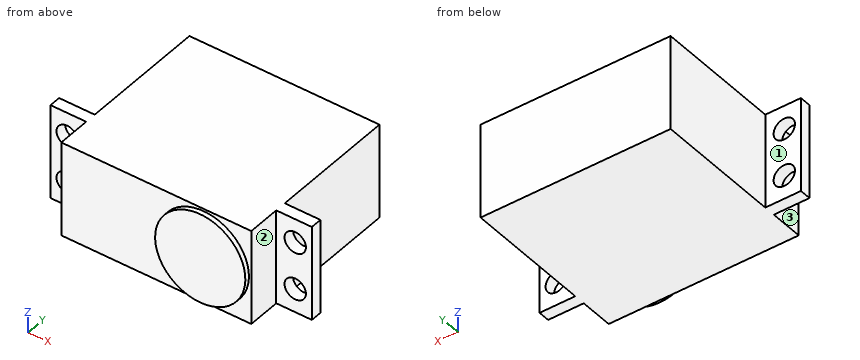
from build123d import *

# Parameters (mm, degrees)
SKETCH1_W            = 40
SKETCH1_H            = 20
BOSS_EXTRUDE1_DEPTH  = 36
SKETCH2_W            = 55
SKETCH2_H            = 20
BOSS_EXTRUDE2_DEPTH  = 2.4
M4_CLEARANCE_HOLE1_D = 4.5
SKETCH5_R            = 9.5
BOSS_EXTRUDE3_DEPTH  = 1


with BuildPart() as part:
    # Sketch1 → Boss-Extrude1 (new body)
    with BuildSketch(Plane(origin=(0, 0, 0), x_dir=(1, 0, 0), z_dir=(0, 1, 0))):
        Rectangle(SKETCH1_W, SKETCH1_H)
    extrude(amount=BOSS_EXTRUDE1_DEPTH)

    # Sketch2 → Boss-Extrude2 (add)
    with BuildSketch(Plane(origin=(0, 7, 0), x_dir=(1, 0, 0), z_dir=(0, 1, 0))):
        Rectangle(SKETCH2_W, SKETCH2_H)
    extrude(amount=BOSS_EXTRUDE2_DEPTH)

    # M4 Clearance Hole1 (through all)
    with Locations(Plane(origin=(0, 7, 0), x_dir=(-1, 0, 0), z_dir=(0, -1, 0))):
        with Locations((-24, 5), (-24, -5)):
            m4_clearance_hole1 = Hole(M4_CLEARANCE_HOLE1_D / 2)

    # Mirror1: M4 Clearance Hole1 across plane
    add(m4_clearance_hole1.mirror(Plane(origin=(0, 0, 0), x_dir=(0, 0, 1), z_dir=(1, 0, 0))), mode=Mode.SUBTRACT)

    # Sketch5 → Boss-Extrude3 (add)
    with BuildSketch(Plane.XZ):
        with Locations(Location((10, 0, 0), (0, 0, 270))):
            Circle(SKETCH5_R)
    extrude(amount=BOSS_EXTRUDE3_DEPTH)


solid = part.part
For this review, take the finished solid that the model builds, in its own axes (mm). Face numbers are marked on the shaded views. A direction names the side the tool comes from. Give positions to 0.01 mm unless a question says otherwise; leave off trailing zeros. Loops run counter-clockwise (first coordinate to the right, second up) from the corner with the lowest first, then second, coordinate; pieces in that order, holes last. Notation, with made-up numbers: M -22,-1.75 L 32,-1.75 A22 ccw 32,5.25 Z; hole C 80,51.5 d3. An arc over 180 degrees is marked long. Put each result on its own line as item: value. Start each with the question number.
(1) Add section C-C, the plane z = 0.25. Write out the cut boundary in (x, y).
(2) Add section A-A, the plane x = -24. Write out the cut boundary in (y, z).
(3) For pin 1 (1 mm diameter, centred on y = 30.5, z = -3.5, fed in from -X); pin 2 (6 mm diameter, centred on x = 24.5, z = 3, fed in from +Y); pin 3 (3.5 mm diameter, centred on x = 24, z = 5, fed in from +Y); pin 4 (8 mm diameter, centred on y = 20, z = 3, fed in from +X), all flat-tipped, find the tip position at first contact; note any pin that passes through.
(4) Machinability: for the marked faces 1, 2 and 3, which of the approach directions +Z, -Z, +X, -X, +Y, -Y give a long, thin tool a straight path to every point of the face, cutting with its end or side? Answer none if there is none.
(5) Add section B-B, the plane z = -5. Write out the cut boundary in (x, y).
(6) Add section D-D, the plane y = 21.5. Write out the cut boundary in (x, z), then the cut area to 3 significant figures.
(7) Wall thickness on L1, parallel to Z at x = -24, y = 8.3; L2, parallel to Y at x = -4, z = 2; L3, parallel to Y at x = 22.5, z = 8.75: over which ranges is each line inside the solid? List them lowest first.
Result:
1. outline: M -27.5,7 L -20,7 L -20,0 L 0.5,0 L 0.5,-1 L 19.5,-1 L 19.5,0 L 20,0 L 20,7 L 27.5,7 L 27.5,9.4 L 20,9.4 L 20,36 L -20,36 L -20,9.4 L -27.5,9.4 Z
2. outline: M 7,-10 L 9.4,-10 L 9.4,-7.25 L 7,-7.25 Z; M 7,-2.75 L 9.4,-2.75 L 9.4,2.75 L 7,2.75 Z; M 7,7.25 L 9.4,7.25 L 9.4,10 L 7,10 Z
3. pin 1: stops at x = -20
3. pin 2: stops at y = 9.4
3. pin 3: passes through
3. pin 4: stops at x = 20
4. face 1: +Z, -Z, -X, +Y
4. face 2: +Z, -Z, +X, -Y
4. face 3: +Z, -Z, -X, -Y
5. outline: M -27.5,7 L -26.25,7 L -26.25,9.4 L -27.5,9.4 Z; M -21.75,7 L -20,7 L -20,0 L 1.92,0 L 1.92,-1 L 18.08,-1 L 18.08,0 L 20,0 L 20,7 L 21.75,7 L 21.75,9.4 L 20,9.4 L 20,36 L -20,36 L -20,9.4 L -21.75,9.4 Z; M 26.25,7 L 27.5,7 L 27.5,9.4 L 26.25,9.4 Z
6. outline: M -20,-10 L 20,-10 L 20,10 L -20,10 Z
6. area: 800 mm^2
7. L1: z = -10 to -7.25, -2.75 to 2.75, 7.25 to 10
7. L2: y = 0 to 36
7. L3: y = 7 to 9.4
